Could you check a few things on this model? Use its own coordinates, in mm. A direction names the side the tool comes from. Give positions to 0.01 mm unless a question says otherwise; leave off trailing zeros. Loops run counter-clockwise (first coordinate to the right, second up) from the corner with the lowest first, then second, coordinate; pieces in that order, holes last. Notation, with made-up numbers: (54, -5.5) - (62, -5.5) arc R14 ccw to (62, 2.5) - close; hole circle Ø1 at (-24.5, -21.5). An arc over 180 degrees is marked (long way). One line per item, written item: value. Start each with the question number.
Q1. If we mould it in two halves opening along Z, with no side actions, what happens to faces 5 (the face through (-64, 18, 0)), 6 (the face through (-64, 17, 0)), 7 (the face through (-1, 3, -8))? For each: released by +Z, released by -Z, zero draft, split by the parting line, or undercut.
Q2. I want a section at B-B (y = 15). Please give me the cut outline in (x, z), then the cut area to 3 significant figures.
Q3. I want a section at A-A (x = -10). Please give me the cut outline in (y, z), then the cut area to 3 significant figures.
Q4. If I drill on line 1 (Z direction, x = 10, y = 4.05); line 2 (X direction, y = 14.5, z = 7.25); line 3 (Y direction, x = -63.5, z = 0), over which ranges is the centre line in solid material (lowest first)? Write a range as from..to.
Q5. I want a section at D-D (z = 0). Count the separate pieces of the cut face and the enclosed holes in it, then the cut area to 3 significant figures.
Q6. I'm going to push flat-ended pins straight in: P1, Ø2, axis at x = -38, y = 9.5, coming from the +Z side; P2, Ø3.5, axis at x = 26, z = 6.5, coming from the +Y side; P3, Ø6.5, axis at x = -42, z = 0, coming from the -Y side. Where does each tip first touch, or does it pass through?
Q7. For faces 1 (the face through (65, 11, 0)), 2 (the face through (-1, 7, 5)), 3 (the face through (-1, 8, 6)), 4 (the face through (-40, 2, -1)), which set-ups out of +Z, -Z, +X, -X, +Y, -Y let a thin tool reach every point of the face, with its end or its side?
Q8. I want a section at C-C (x = 48.5). Please give me the cut outline in (y, z), then the cut area to 3 significant figures.
```python
from build123d import *

# Parameters (mm, degrees)
SKETCH1_W               = 130
SKETCH1_H               = 16
BOSS_EXTRUDE1_DEPTH     = 5
SKETCH2_W               = 130
SKETCH2_H               = 16
SKETCH2_W_2             = 124
SKETCH2_H_2             = 10
BOSS_EXTRUDE2_DEPTH     = 3
SKETCH3_W               = 3
SKETCH3_H               = 16
BOSS_EXTRUDE3_DEPTH     = 10
FILLET1_R               = 4
SKETCH4_R               = 2
CUT_EXTRUDE1_DEPTH      = 10
SKETCH6_R               = 4
CUT_EXTRUDE2_DEPTH      = 2
SKETCH7_R               = 2
CUT_EXTRUDE3_DEPTH      = 5
CUT_EXTRUDE4_DEPTH      = 129.518481161
CUT_EXTRUDE4_DEPTH_BACK = 129.518481161
SKETCH8_R               = 2


with BuildPart() as part:
    # Sketch1 → Boss-Extrude1 (new body)
    with BuildSketch(Plane(origin=(0, 0, 0), x_dir=(1, 0, 0), z_dir=(0, 1, 0))):
        Rectangle(SKETCH1_W, SKETCH1_H)
    extrude(amount=BOSS_EXTRUDE1_DEPTH)

    # Sketch2 → Boss-Extrude2 (add)
    with BuildSketch(Plane(origin=(0, 5, 0), x_dir=(1, 0, 0), z_dir=(0, 1, 0))):
        Rectangle(SKETCH2_W, SKETCH2_H)
        Rectangle(SKETCH2_W_2, SKETCH2_H_2, mode=Mode.SUBTRACT)
    extrude(amount=BOSS_EXTRUDE2_DEPTH)

    # Sketch3 → Boss-Extrude3 (add)
    with BuildSketch(Plane(origin=(0, 8, 0), x_dir=(1, 0, 0), z_dir=(0, 1, 0))):
        with Locations((-63.5, 0)):
            Rectangle(SKETCH3_W, SKETCH3_H)
        with Locations((63.5, 0)):
            Rectangle(SKETCH3_W, SKETCH3_H)
    extrude(amount=BOSS_EXTRUDE3_DEPTH)

    # Fillet1
    fillet1_edges = [part.edges().sort_by_distance(p)[0] for p in [
        (-62, 8, -6.5),
        (-62, 8, 6.5),
        (62, 8, -6.5),
        (62, 8, 6.5),
    ]]
    fillet(fillet1_edges, radius=FILLET1_R)

    # Sketch4 → Cut-Extrude1 (cut)
    with BuildSketch(Plane(origin=(0, 5, 0), x_dir=(1, 0, 0), z_dir=(0, 1, 0))):
        with Locations(Location((42, 0, 0), (0, 0, 270))):
            Circle(SKETCH4_R)
        with Locations(Location((-42, 0, 0), (0, 0, 270))):
            Circle(SKETCH4_R)
    extrude(amount=-CUT_EXTRUDE1_DEPTH, mode=Mode.SUBTRACT)

    # Sketch6 → Cut-Extrude2 (cut)
    with BuildSketch(Plane.XZ):
        with Locations(Location((42, 0, 0), (0, 0, 270))):
            Circle(SKETCH6_R)
        with Locations(Location((-42, 0, 0), (0, 0, 270))):
            Circle(SKETCH6_R)
    extrude(amount=-CUT_EXTRUDE2_DEPTH, mode=Mode.SUBTRACT)

    # Sketch7 → Cut-Extrude3 (cut)
    with BuildSketch(Plane(origin=(0, 5, 0), x_dir=(1, 0, 0), z_dir=(0, 1, 0))):
        with Locations(Location((0, 0, 0), (0, 0, 270))):
            Circle(SKETCH7_R)
        with Locations(Location((-10, 0, 0), (0, 0, 270))):
            Circle(SKETCH7_R)
        with Locations(Location((-20, 0, 0), (0, 0, 270))):
            Circle(SKETCH7_R)
        with Locations(Location((-30, 0, 0), (0, 0, 270))):
            Circle(SKETCH7_R)
        with Locations(Location((-54.066395838, 0, 0), (0, 0, 270))):
            Circle(SKETCH7_R)
        with Locations(Location((54.066395838, 0, 0), (0, 0, 90))):
            Circle(SKETCH7_R)
        with Locations(Location((30, 0, 0), (0, 0, 90))):
            Circle(SKETCH7_R)
        with Locations(Location((20, 0, 0), (0, 0, 90))):
            Circle(SKETCH7_R)
        with Locations(Location((10, 0, 0), (0, 0, 90))):
            Circle(SKETCH7_R)
    extrude(amount=-CUT_EXTRUDE3_DEPTH, mode=Mode.SUBTRACT)

    # Sketch8 → Cut-Extrude4 (cut, two sides: drawn at the far end of the back side and taken through both)
    with BuildSketch(Plane(origin=(-62, 0, 0), x_dir=(0, 0, -1), z_dir=(1, 0, 0)).offset(-CUT_EXTRUDE4_DEPTH_BACK)):
        with Locations((0, 8.5)):
            Circle(SKETCH8_R)
        with Locations((0, 15)):
            Circle(SKETCH8_R)
    extrude(amount=CUT_EXTRUDE4_DEPTH + CUT_EXTRUDE4_DEPTH_BACK, mode=Mode.SUBTRACT)


solid = part.part
```
Worked answers:
1. face 5: zero draft
1. face 6: undercut
1. face 7: released by -Z
2. outline: (-65, -8) - (-62, -8) - (-62, -2) - (-65, -2) - close; (-65, 2) - (-62, 2) - (-62, 8) - (-65, 8) - close; (62, -8) - (65, -8) - (65, -2) - (62, -2) - close; (62, 2) - (65, 2) - (65, 8) - (62, 8) - close
2. area: 72.0 mm²
3. outline: (0, -8) - (8, -8) - (8, -5) - (5, -5) - (5, -2) - (0, -2) - close; (0, 2) - (5, 2) - (5, 5) - (8, 5) - (8, 8) - (0, 8) - close
3. area: 78.0 mm²
4. line 1: z = -8..-2, 2..8
4. line 2: x = -65..-62, 62..65
4. line 3: y = 0..6.5, 10.5..13, 17..18
5. separate pieces: 16
5. enclosed holes: 0
5. area: 444 mm²
6. P1: passes through
6. P2: stops at y = 8
6. P3: stops at y = 2
7. face 1: +Z, -Z, +X, +Y, -Y
7. face 2: +Y
7. face 3: +Z, -Z, +Y
7. face 4: -Y
8. outline: (0, -8) - (8, -8) - (8, -5) - (5, -5) - (5, 5) - (8, 5) - (8, 8) - (0, 8) - close
8. area: 98.0 mm²
